Can you work these out from the model? Positions are in its coordinate system, mm. Face numbers are marked on the shaded views. A direction names the side the tool comes from. Round coordinates to 2 decimals unless told otherwise and drop trailing zeros. Write each loop counter-clockwise with the first axis right and the second up, starting at its lowest first coordinate (ties: lowest second). Pieces come first, ordered by that corner, then holes.
Q1. For the marked faces 5, 6, 7 and 8, which set-ups out of +Z, -Z, +X, -X, +Y, -Y let a thin tool reach every point of the face, with its end or its side?
Q2. If we section it at D-D (y = -8.5): Please give me the cut outline in (x, z) (1 decimal).
Q3. If we section it at A-A (z = 8.75): Please give me the cut outline in (x, y), plus the area to 3 significant figures.
Q4. Please list where these lines run through material, in increasing order: line 1 along X through (y, z) = (-8.5, 6.25) (1 decimal); line 2 along X through (y, z) = (30, 4).
Q5. We'd pull the mould along X, two halves only. Please class the marked faces 1, 2, 3 and 4: +X half, -X half, draft (parallel to the pull), parting line (faces both ways), or undercut.
Q6. If we section it at C-C (x = -25.5): Please give me the cut outline in (y, z), plus the area to 3 significant figures.
Q7. I'm going to push flat-ended pins straight in: pin 1 Ø0.5 at (x, y) = (-22, 8) entering from -Z; pin 2 Ø4 at (y, z) = (22.5, -3) entering from -X; pin 3 Ø3 at (x, z) = (-32, 0) entering from +Y; pin 4 Ø12.5 at (x, z) = (4, -2) entering from +Y. Where does each tip first touch, or does it pass through?
Q8. If we section it at B-B (y = 27): Please give me the cut outline in (x, z), plus the area to 3 significant figures.
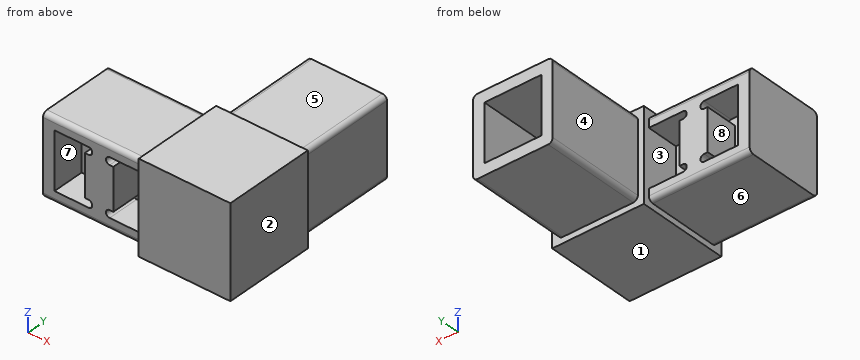
from build123d import *

# Parameters (mm, degrees)
SKETCH1_W           = 25.4
SKETCH1_H           = 22.098
BOSS_EXTRUDE1_DEPTH = 1.651
SKETCH2_W           = 53.34
SKETCH2_H           = 22.098
BOSS_EXTRUDE2_DEPTH = 22.098
SKETCH3_W           = 25.4
SKETCH3_H           = 22.098
BOSS_EXTRUDE3_DEPTH = 1.651
SKETCH4_W           = 25.4
SKETCH4_H           = 25.4
BOSS_EXTRUDE4_DEPTH = 1.651
SKETCH5_W           = 25.4
SKETCH5_H           = 25.4
BOSS_EXTRUDE5_DEPTH = 1.651
CUT_EXTRUDE1_DEPTH  = 8.89
CUT_EXTRUDE2_DEPTH  = 8.89
CUT_EXTRUDE3_DEPTH  = 8.89
CUT_EXTRUDE4_DEPTH  = 8.89
SKETCH10_W          = 22.098
SKETCH10_H          = 22.098
BOSS_EXTRUDE6_DEPTH = 27.94
SKETCH11_W          = 15.748
SKETCH11_H          = 15.748
CUT_EXTRUDE5_DEPTH  = 27.94
FILLET1_R           = 1.27


with BuildPart() as part:
    # Sketch1 → Boss-Extrude1 (new body)
    with BuildSketch(Plane(origin=(0, 0, -12.7), x_dir=(-1, 0, 0), z_dir=(0, 0, -1))):
        Rectangle(SKETCH1_W, SKETCH1_H)
    extrude(amount=-BOSS_EXTRUDE1_DEPTH)

    # Sketch2 → Boss-Extrude2 (add)
    with BuildSketch(Plane.XY.offset(-11.049)):
        with Locations((-13.97, 0)):
            Rectangle(SKETCH2_W, SKETCH2_H)
    extrude(amount=BOSS_EXTRUDE2_DEPTH)

    # Sketch3 → Boss-Extrude3 (add)
    with BuildSketch(Plane.XY.offset(11.049)):
        Rectangle(SKETCH3_W, SKETCH3_H)
    extrude(amount=BOSS_EXTRUDE3_DEPTH)

    # Sketch4 → Boss-Extrude4 (add)
    with BuildSketch(Plane(origin=(0, 11.049, 0), x_dir=(-1, 0, 0), z_dir=(0, 1, 0))):
        Rectangle(SKETCH4_W, SKETCH4_H)
    extrude(amount=BOSS_EXTRUDE4_DEPTH)

    # Sketch5 → Boss-Extrude5 (add)
    with BuildSketch(Plane.XZ.offset(11.049)):
        Rectangle(SKETCH5_W, SKETCH5_H)
    extrude(amount=BOSS_EXTRUDE5_DEPTH)

    # Sketch6 → Cut-Extrude1 (cut)
    with BuildSketch(Plane(origin=(0, 11.049, 0), x_dir=(-1, 0, 0), z_dir=(0, 1, 0))):
        with BuildLine():
            Line((21.1455, 5.842), (22.1615, 5.842))
            ThreePointArc((22.1615, 5.842), (23.1775, 6.858), (22.1615, 7.874))
            Line((22.1615, 7.874), (12.7, 7.874))
            Line((12.7, 7.874), (12.7, -7.874))
            Line((12.7, -7.874), (22.1615, -7.874))
            ThreePointArc((22.1615, -7.874), (23.1775, -6.858), (22.1615, -5.842))
            Line((22.1615, -5.842), (21.1455, -5.842))
            Line((21.1455, -5.842), (21.1455, 5.842))
        make_face()
    extrude(amount=-CUT_EXTRUDE1_DEPTH, mode=Mode.SUBTRACT)

    # Sketch7 → Cut-Extrude2 (cut)
    with BuildSketch(Plane.XZ.offset(11.049)):
        with BuildLine():
            Line((-22.1615, 5.842), (-21.1455, 5.842))
            Line((-21.1455, 5.842), (-21.1455, -5.842))
            Line((-21.1455, -5.842), (-22.1615, -5.842))
            ThreePointArc((-22.1615, -5.842), (-23.1775, -6.858), (-22.1615, -7.874))
            Line((-22.1615, -7.874), (-12.7, -7.874))
            Line((-12.7, -7.874), (-12.7, 7.874))
            Line((-12.7, 7.874), (-22.1615, 7.874))
            ThreePointArc((-22.1615, 7.874), (-23.1775, 6.858), (-22.1615, 5.842))
        make_face()
    extrude(amount=-CUT_EXTRUDE2_DEPTH, mode=Mode.SUBTRACT)

    # Sketch8 → Cut-Extrude3 (cut)
    with BuildSketch(Plane(origin=(0, 11.049, 0), x_dir=(-1, 0, 0), z_dir=(0, 1, 0))):
        with BuildLine():
            Line((28.0035, -7.874), (37.465, -7.874))
            Line((37.465, -7.874), (37.465, 7.874))
            Line((37.465, 7.874), (28.0035, 7.874))
            ThreePointArc((28.0035, 7.874), (26.9875, 6.858), (28.0035, 5.842))
            Line((28.0035, 5.842), (29.0195, 5.842))
            Line((29.0195, 5.842), (29.0195, -5.842))
            Line((29.0195, -5.842), (28.0035, -5.842))
            ThreePointArc((28.0035, -5.842), (26.9875, -6.858), (28.0035, -7.874))
        make_face()
    extrude(amount=-CUT_EXTRUDE3_DEPTH, mode=Mode.SUBTRACT)

    # Sketch9 → Cut-Extrude4 (cut)
    with BuildSketch(Plane.XZ.offset(11.049)):
        with BuildLine():
            Line((-37.465, 7.874), (-37.465, -7.874))
            Line((-37.465, -7.874), (-28.0035, -7.874))
            ThreePointArc((-28.0035, -7.874), (-26.9875, -6.858), (-28.0035, -5.842))
            Line((-28.0035, -5.842), (-29.0195, -5.842))
            Line((-29.0195, -5.842), (-29.0195, 5.842))
            Line((-29.0195, 5.842), (-28.0035, 5.842))
            ThreePointArc((-28.0035, 5.842), (-26.9875, 6.858), (-28.0035, 7.874))
            Line((-28.0035, 7.874), (-37.465, 7.874))
        make_face()
    extrude(amount=-CUT_EXTRUDE4_DEPTH, mode=Mode.SUBTRACT)

    # Sketch10 → Boss-Extrude6 (add)
    with BuildSketch(Plane(origin=(0, 12.7, 0), x_dir=(-1, 0, 0), z_dir=(0, 1, 0))):
        Rectangle(SKETCH10_W, SKETCH10_H)
    extrude(amount=BOSS_EXTRUDE6_DEPTH)

    # Sketch11 → Cut-Extrude5 (cut)
    with BuildSketch(Plane(origin=(0, 40.64, 0), x_dir=(-1, 0, 0), z_dir=(0, 1, 0))):
        Rectangle(SKETCH11_W, SKETCH11_H)
    extrude(amount=-CUT_EXTRUDE5_DEPTH, mode=Mode.SUBTRACT)

    # Fillet1
    fillet1_edges = [part.edges().sort_by_distance(p)[0] for p in [
        (-26.67, 11.049, -11.049),
        (-26.67, -11.049, -11.049),
        (-26.67, -11.049, 11.049),
        (-11.049, 26.67, -11.049),
        (-11.049, 26.67, 11.049),
        (11.049, 26.67, 11.049),
        (11.049, 26.67, -11.049),
        (-26.67, 11.049, 11.049),
    ]]
    fillet(fillet1_edges, radius=FILLET1_R)


solid = part.part
A:
1. face 5: +Z, +X, -X, +Y
1. face 6: -Z, -X, +Y, -Y
1. face 7: -Y
1. face 8: +Y
2. outline: (-40.6, -11) - (-12.7, -11) - (-12.7, -12.7) - (12.7, -12.7) - (12.7, 12.7) - (-12.7, 12.7) - (-12.7, 11) - (-40.6, 11) - close; hole (-37.5, -7.9) - (-28, -7.9) arc R1 ccw to (-28, -5.8) - (-29, -5.8) - (-29, 5.8) - (-28, 5.8) arc R1 ccw to (-28, 7.9) - (-37.5, 7.9) - close; hole (-22.2, -7.9) - (-12.7, -7.9) - (-12.7, 7.9) - (-22.2, 7.9) arc R1 ccw to (-22.2, 5.8) - (-21.1, 5.8) - (-21.1, -5.8) - (-22.2, -5.8) arc R1 ccw to start
3. outline: (-40.64, -11.05) - (-12.7, -11.05) - (-12.7, -12.7) - (12.7, -12.7) - (12.7, 12.7) - (11.05, 12.7) - (11.05, 40.64) - (-11.05, 40.64) - (-11.05, 12.7) - (-12.7, 12.7) - (-12.7, 11.05) - (-40.64, 11.05) - close
3. area: 1,880 mm2
4. line 1: x = -40.6 to -37.5, -27.2 to -23, -12.7 to 12.7
4. line 2: x = -11.05 to -7.87, 7.87 to 11.05
5. face 1: draft
5. face 2: +X half
5. face 3: undercut
5. face 4: -X half
6. outline: (-11.05, -9.78) arc R1.27 ccw to (-9.78, -11.05) - (9.78, -11.05) arc R1.27 ccw to (11.05, -9.78) - (11.05, 9.78) arc R1.27 ccw to (9.78, 11.05) - (-9.78, 11.05) arc R1.27 ccw to (-11.05, 9.78) - close
6. area: 487 mm2
7. pin 1: stops at z = -11.05
7. pin 2: stops at x = -11.05
7. pin 3: stops at y = 2.16
7. pin 4: stops at y = 40.64
8. outline: (-11.05, -9.78) arc R1.27 ccw to (-9.78, -11.05) - (9.78, -11.05) arc R1.27 ccw to (11.05, -9.78) - (11.05, 9.78) arc R1.27 ccw to (9.78, 11.05) - (-9.78, 11.05) arc R1.27 ccw to (-11.05, 9.78) - close; hole (-7.87, -7.87) - (7.87, -7.87) - (7.87, 7.87) - (-7.87, 7.87) - close
8. area: 239 mm2
